Job drawing, mm, ordinate dimensions from the low corner. One solid piece. Round coordinates to 2 decimals unless told otherwise and drop trailing zeros. Write each loop counter-clockwise with the first axis right and the second up, starting at its lowest first coordinate (ties: lowest second). Pieces come first, ordered by that corner, then holes. Notation, with made-up numbers: M 8.5,12 L 34.5,12 A23 cw 34.5,37 Z; hole C -9,-5.75 d8. An arc over 180 degrees is marked long. One line per item, written item: value. Start each with the question number.
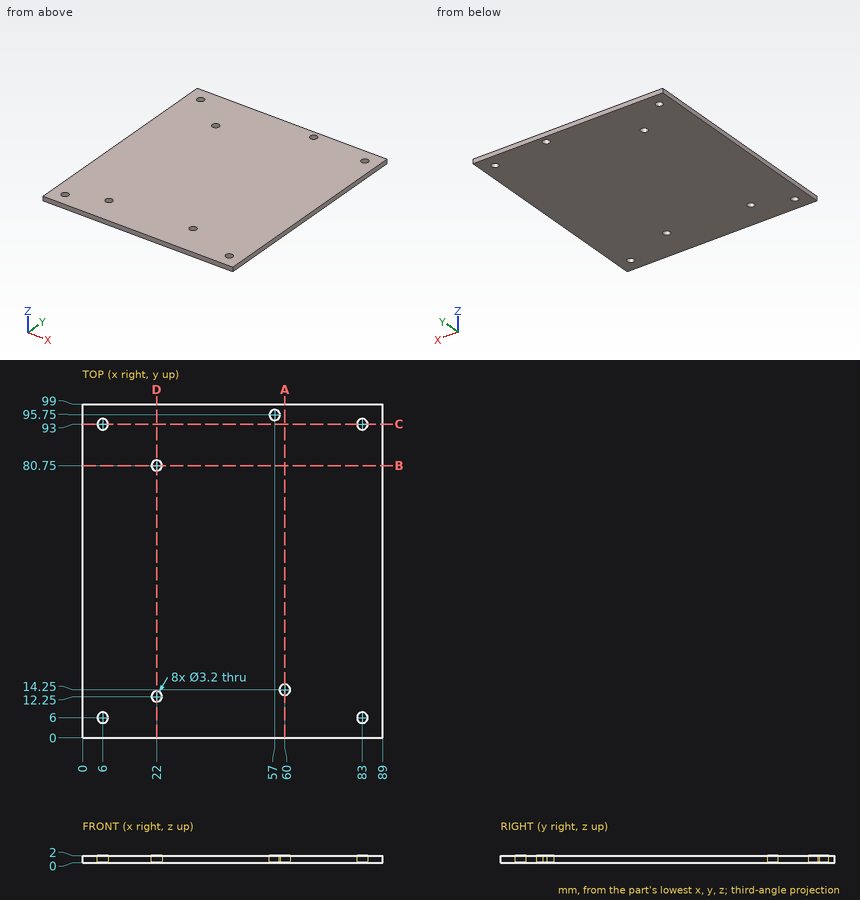
Item 1: Cut at D-D, the plane x = 22. Write the cut outline in (y, z), plus the area to 3 significant figures.
Item 2: Cut at B-B, the plane y = 80.75. Write the cut outline in (x, z).
Item 3: Cut at C-C, the plane y = 93. Write the cut outline in (x, z), plus the area to 3 significant figures.
Item 4: Drill centre lines: line 1 (X direction, y = 93, z = 1.4); line 2 (Y direction, x = 6, z = 0.7); line 3 (X direction, y = 14.5, z = 1.75). Where is each one in solid material? Low to high.
Item 5: Cut at A-A, the plane x = 60. Write the cut outline in (y, z).
Computed values:
1. outline: M 0,0 L 10.65,0 L 10.65,2 L 0,2 Z; M 13.85,0 L 79.15,0 L 79.15,2 L 13.85,2 Z; M 82.35,0 L 99,0 L 99,2 L 82.35,2 Z
1. area: 185 mm2
2. outline: M 0,0 L 20.4,0 L 20.4,2 L 0,2 Z; M 23.6,0 L 89,0 L 89,2 L 23.6,2 Z
3. outline: M 0,0 L 4.4,0 L 4.4,2 L 0,2 Z; M 7.6,0 L 81.4,0 L 81.4,2 L 7.6,2 Z; M 84.6,0 L 89,0 L 89,2 L 84.6,2 Z
3. area: 165 mm2
4. line 1: x = 0 to 4.4, 7.6 to 81.4, 84.6 to 89
4. line 2: y = 0 to 4.4, 7.6 to 91.4, 94.6 to 99
4. line 3: x = 0 to 58.42, 61.58 to 89
5. outline: M 0,0 L 12.65,0 L 12.65,2 L 0,2 Z; M 15.85,0 L 99,0 L 99,2 L 15.85,2 Z
